For this review, take the finished solid that the model builds, in its own axes (mm). A direction names the side the tool comes from. Round coordinates to 2 decimals unless told otherwise and drop trailing zeros. Write each loop counter-clockwise with the first axis right and the second up, starting at its lowest first coordinate (ties: lowest second). Pieces come first, ordered by that corner, then holes. Notation, with made-up numbers: M -19,58 L 28,58 A19 cw 28,77 Z; hole C 6,50 d11. An arc over 180 degrees is marked long. Use one line per item in the form item = value. Start each with the question number.
Item 1: Add section A-A (z = 100). State the section outline as (x, y) points, and give its area (3 significant figures).
Item 2: For line 1 (Z direction, x = 62, y = -10); line 2 (X direction, y = -20, z = 104.5); line 3 (Z direction, x = 64.6, y = -10), list the stretches that pass through material, from the lowest coordinate up. Write a range as [from, to].
Item 3: For P1, Ø4.5, axis at x = 108, z = 46, coming from the -Y side; P2, Ø8.5, axis at y = -10, z = 100, coming from the -X side; P3, Ø16.5, axis at y = -11, z = 107, coming from the +X side; P4, Ø6, axis at y = -10, z = 120, coming from the +X side, all flat-tipped, find the tip position at first contact; note any pin that passes through.
Item 4: For faces 1 (the flat face through (115, -9.192, 31)), 2 (the flat face through (106, -13.268, 44)), 3 (the cylindrical face through (95.783, -16.724, 59.195)), list the 3-axis set-ups (+Z, -Z, +X, -X, +Y, -Y) from which the entire face can be reached by the end or side of a thin tool; tool diameter is ignored.
Item 5: Draft analysis for pull direction Y (two halves, no side actions). For faces 4 (the cylindrical face through (99.252, -0.285, 55.303)), 5 (the flat face through (96, -7.397, 59)), 6 (the flat face through (69, -17, 10)), state which applies: released by +Y, released by -Y, zero draft, split by the parting line, or undercut.
Item 6: Add section B-B (y = -23.5). State the section outline as (x, z) points.
from build123d import *

# Parameters (mm, degrees)
F0_W      = 110
F0_H      = 20
F1_DEPTH  = 35
F2_W      = 3.4
F2_H      = 70
F3_DEPTH  = 30
F4_R      = 3.25
F5_DEPTH  = 25
F7_DEPTH  = 35.001
F8_R      = 5
F9_R      = 3
F10_R     = 5
F11_R     = 1
F12_R     = 1
F13_R     = 1
F15_DEPTH = 2


with BuildPart() as f1:
    # F0 (on Front) → F1 (new body)
    with BuildSketch(Plane.XZ):
        with Locations((68.5714285714, 10)):
            Rectangle(F0_W, F0_H)
        Polygon((61.0714285714, 90), (13.5714285714, 20), (123.5714285714, 20), (76.0714285714, 90), align=None)
        Polygon((68.5714285714, 101.0526315789), (61.0714285714, 90), (76.0714285714, 90), align=None)
        Polygon((61.0714285714, 150), (61.0714285714, 90), (68.5714285714, 101.0526315789), (76.0714285714, 90), (76.0714285714, 150), align=None)
    extrude(amount=F1_DEPTH)

    # F2 (on face) → F3 (cut)
    with BuildSketch(Plane(origin=(0, 0, 0), x_dir=(-1, 0, 0), z_dir=(0, 1, 0))):
        with Locations((-68.5714285714, 115)):
            Rectangle(F2_W, F2_H)
    extrude(amount=-F3_DEPTH, mode=Mode.SUBTRACT)

    # F4 (on face) → F5 (cut)
    with BuildSketch(Plane.YZ.offset(76.0714285714)):
        with Locations((-10, 140)):
            Circle(F4_R)
        with Locations((-10, 120)):
            Circle(F4_R)
        with Locations((-10, 100)):
            Circle(F4_R)
    extrude(amount=-F5_DEPTH, mode=Mode.SUBTRACT)

    # F6 (on face) → F7 (cut, through all)
    with BuildSketch(Plane(origin=(0, 0, 0), x_dir=(-1, 0, 0), z_dir=(0, 1, 0))):
        Polygon((-71.5154382332, 70), (-112.2297239475, 10), (-24.9131331954, 10), (-65.6274189097, 70), align=None)
    extrude(amount=-F7_DEPTH, mode=Mode.SUBTRACT)

    # F8
    f8_edges = [f1.edges().sort_by_distance(p)[0] for p in [
        (24.913133, -17.5, 10),
        (112.229724, -17.5, 10),
        (13.571429, -17.5, 20),
        (123.571429, -17.5, 20),
        (61.071429, -17.5, 90),
        (76.071429, -17.5, 90),
    ]]
    fillet(f8_edges, radius=F8_R)

    # F9
    f9_edges = [f1.edges().sort_by_distance(p)[0] for p in [
        (71.515438, -17.5, 70),
        (65.627419, -17.5, 70),
    ]]
    fillet(f9_edges, radius=F9_R)

    # F10
    f10_edges = [f1.edges().sort_by_distance(p)[0] for p in [
        (73.171429, 0, 150),
        (63.971429, 0, 150),
    ]]
    fillet(f10_edges, radius=F10_R)

    # F11
    f11_edges = [f1.edges().sort_by_distance(p)[0] for p in [
        (76.071429, -35, 120.768138),
        (61.071429, -35, 120.768138),
    ]]
    fillet(f11_edges, radius=F11_R)

    # F12
    f12_edges = [f1.edges().sort_by_distance(p)[0] for p in [
        (68.571429, -35, 150),
    ]]
    fillet(f12_edges, radius=F12_R)

    # F13
    f13_edges = [f1.edges().sort_by_distance(p)[0] for p in [
        (47.472923, 0, 43.246006),
        (47.472923, -35, 43.246006),
    ]]
    fillet(f13_edges, radius=F13_R)

    # F14 (on face) → F15 (cut)
    with BuildSketch(Plane(origin=(93.903930131, 0, 63.7205240175), x_dir=(0, 1, 0), z_dir=(0.8274757744, 0, 0.5615014183))):
        with BuildLine():
            ThreePointArc((-7.39691, -42.389428057), (-7.5085023164, -42.6588357407), (-7.77791, -42.770428057))
            Line((-7.77791, -42.770428057), (-9.19156, -42.770428057))
            Line((-9.19156, -42.770428057), (-9.19156, -33.770818057))
            ThreePointArc((-9.19156, -33.770818057), (-10.33456, -32.627818057), (-11.47756, -33.770818057))
            Line((-11.47756, -33.770818057), (-11.47756, -42.907248057))
            ThreePointArc((-11.47756, -42.907248057), (-11.1260881374, -43.7557761945), (-10.27756, -44.107248057))
            Line((-10.27756, -44.107248057), (-7.3415622471, -44.107248057))
            ThreePointArc((-7.3415622471, -44.107248057), (-5.9934152346, -43.7495106005), (-5, -42.770428057))
            Line((-5, -42.770428057), (-5, -21.7097182665))
            ThreePointArc((-5, -21.7097182665), (-8.1953654076, -19.9118808439), (-11.47756, -21.5458264194))
            Line((-11.47756, -21.5458264194), (-11.47756, -29.7319929648))
            ThreePointArc((-11.47756, -29.7319929648), (-12.3791235209, -30.0442725829), (-13.26801, -29.6975505479))
            Line((-13.26801, -29.6975505479), (-13.26801, -17.3213335826))
            ThreePointArc((-13.26801, -17.3213335826), (-12.3963505956, -17.6932012527), (-11.45723, -17.820198057))
            Line((-11.45723, -17.820198057), (-5.85734, -17.820198057))
            ThreePointArc((-5.85734, -17.820198057), (-4.99482, -16.957678057), (-5.85734, -16.095158057))
            Line((-5.85734, -16.095158057), (-11.45723, -16.095158057))
            ThreePointArc((-11.45723, -16.095158057), (-12.7376448172, -15.5647928743), (-13.26801, -14.284378057))
            Line((-13.26801, -14.284378057), (-13.26801, -11.295158057))
            Line((-13.26801, -11.295158057), (-8.99429, -11.295158057))
            ThreePointArc((-8.99429, -11.295158057), (-8.3556712039, -11.1905981156), (-7.7837423225, -10.8878373145))
            Line((-7.7837423225, -10.8878373145), (-10.7806342513, -9.578398057))
            Line((-10.7806342513, -9.578398057), (-14.60151, -9.578398057))
            ThreePointArc((-14.60151, -9.578398057), (-15.2750292091, -9.857378848), (-15.55401, -10.530898057))
            Line((-15.55401, -10.530898057), (-15.55401, -29.6749688929))
            ThreePointArc((-15.55401, -29.6749688929), (-12.3872480124, -31.3357744138), (-9.19156, -29.7313322704))
            Line((-9.19156, -29.7313322704), (-9.19156, -21.5494478814))
            ThreePointArc((-9.19156, -21.5494478814), (-8.2941290281, -21.1170780915), (-7.39691, -21.5498875186))
            Line((-7.39691, -21.5498875186), (-7.39691, -42.389428057))
        make_face()
        with BuildLine():
            ThreePointArc((-15.55401, -42.907248057), (-14.41101, -44.050248057), (-13.26801, -42.907248057))
            Line((-13.26801, -42.907248057), (-13.26801, -33.770818057))
            ThreePointArc((-13.26801, -33.770818057), (-14.41101, -32.627818057), (-15.55401, -33.770818057))
            Line((-15.55401, -33.770818057), (-15.55401, -42.907248057))
        make_face()
        with BuildLine():
            Line((-5.4666149713, -8.8973021589), (-14.7725599426, -4.831233057))
            Line((-14.7725599426, -4.831233057), (-5.4666149713, -0.7651639552))
            ThreePointArc((-5.4666149713, -0.7651639552), (-4.9630941019, 0.5198069716), (-6.2480650287, 1.0233278411))
            Line((-6.2480650287, 1.0233278411), (-15.55401, -3.0427412608))
            ThreePointArc((-15.55401, -3.0427412608), (-16.7243199426, -4.831233057), (-15.55401, -6.6197248533))
            Line((-15.55401, -6.6197248533), (-6.2480650287, -10.6857939552))
            ThreePointArc((-6.2480650287, -10.6857939552), (-4.9630941019, -10.1822730857), (-5.4666149713, -8.8973021589))
        make_face()
        with BuildLine():
            ThreePointArc((-9.19156, -6.331233057), (-8.294235, -7.228558057), (-7.39691, -6.331233057))
            Line((-7.39691, -6.331233057), (-7.39691, -3.331233057))
            ThreePointArc((-7.39691, -3.331233057), (-8.294235, -2.433908057), (-9.19156, -3.331233057))
            Line((-9.19156, -3.331233057), (-9.19156, -6.331233057))
        make_face()
        with BuildLine():
            add(Edge.make_bspline(
                [(-19.778765, -10.530898057), (-19.778765, -12.0897437839), (-17.7781475, -11.3103209205), (-15.77753, -10.530898057), (-17.7781475, -9.7514751936), (-19.778765, -8.9720523302), (-19.778765, -10.530898057)],
                knots=[0, 0, 0, 2.0943951024, 2.0943951024, 4.1887902048, 4.1887902048, 6.2831853072, 6.2831853072, 6.2831853072], degree=2, weights=[1, 0.5, 1, 0.5, 1, 0.5, 1]))
        make_face()
    extrude(amount=-F15_DEPTH, mode=Mode.SUBTRACT)


solid = f1.part
Calculated:
q1.outline = M 61.07,-34 A1 ccw 62.07,-35 L 75.07,-35 A1 ccw 76.07,-34 L 76.07,-13.25 L 70.27,-13.25 L 70.27,-30 L 66.87,-30 L 66.87,-13.25 L 61.07,-13.25 Z; M 61.07,-6.75 L 66.87,-6.75 L 66.87,0 L 62.07,0 A1 ccw 61.07,-1 Z; M 70.27,-6.75 L 76.07,-6.75 L 76.07,-1 A1 ccw 75.07,0 L 70.27,0 Z
q1.area = 347 mm^2
q2.line_1 = [0, 10], [64.65, 96.75], [103.25, 116.75], [123.25, 136.75], [143.25, 150]
q2.line_2 = [61.07, 66.87], [70.27, 76.07]
q2.line_3 = [0, 10], [68.49, 96.75], [103.25, 116.75], [123.25, 136.75], [143.25, 150]
q3.P1 = -34.89
q3.P2 = 61.07
q3.P3 = 76.07
q3.P4 = through
q4.face_1 = +X
q4.face_2 = +Z, +X
q4.face_3 = none
q5.face_4 = released by +Y
q5.face_5 = undercut
q5.face_6 = zero draft
q6.outline = M 13.57,0 L 123.57,0 L 123.57,18.46 A5 ccw 122.71,21.27 L 76.93,88.73 A5 cw 76.07,91.54 L 76.07,149 A1 ccw 75.07,150 L 70.27,150 L 70.27,80 L 66.87,80 L 66.87,150 L 62.07,150 A1 ccw 61.07,149 L 61.07,91.54 A5 cw 60.21,88.73 L 14.43,21.27 A5 ccw 13.57,18.46 Z; hole M 30.21,17.81 A5 ccw 34.35,10 L 102.79,10 A5 ccw 106.93,17.81 L 72.41,68.68 A3 ccw 69.93,70 L 67.22,70 A3 ccw 64.73,68.68 Z
